Input: part model. Units: mm. Frame: model coordinates. Face numbers are marked on the shaded views. A direction names the side the tool comes from. Give positions to 0.01 mm unless a question says otherwise; leave off trailing zeros. Loops run counter-clockwise (first coordinate to the right, second up) from the corner with the lowest first, then second, coordinate; pieces in that order, holes last. Notation, with made-up numbers: M -19.75,20 L 32.25,20 A27 ccw 32.25,43 Z; hole C 64.5,75.25 d4. An arc over 180 degrees is marked long. Return JSON: item names as keys, results as strings. Group by question number.
```python
from build123d import *
from build123d import SkipClean  # not in build123d's __all__

# Parameters (mm, degrees)
F4_DEPTH = 10


with BuildPart() as f1:
    # F0 (on Front) → F1 (revolve)
    with BuildSketch(Plane.XZ):
        with BuildLine():
            Line((0, 5), (0, 0))
            Line((0, 0), (17.5, 0))
            Line((17.5, 0), (48.9644660941, 31.4644660941))
            ThreePointArc((48.9644660941, 31.4644660941), (46.4644660941, 32.5), (45.4289321881, 35))
            Line((45.4289321881, 35), (15.4289321881, 5))
            Line((15.4289321881, 5), (0, 5))
        make_face()
        with BuildLine():
            Line((45.4289321881, 35), (52.5, 35))
            ThreePointArc((52.5, 35), (48.9644660941, 38.5355339059), (45.4289321881, 35))
        make_face()
        with BuildLine():
            ThreePointArc((45.4289321881, 35), (46.4644660941, 32.5), (48.9644660941, 31.4644660941))
            Line((48.9644660941, 31.4644660941), (52.5, 35))
            Line((52.5, 35), (45.4289321881, 35))
        make_face()
    revolve(axis=Axis((0, 0, 17.5), (0, 0, 1)))

    # F2 (on face) → F3 (join, up to the next surface of F1)
    with BuildSketch(Plane(origin=(0, 0, 0), x_dir=(1, 0, 0), z_dir=(0, 0, -1))):
        with BuildLine():
            ThreePointArc((17.2839285714, -2.7414983381), (19.3665882743, -2.0194920684), (20.25, 0))
            ThreePointArc((20.25, 0), (19.3665882743, 2.0194920684), (17.2839285714, 2.7414983381))
            ThreePointArc((17.2839285714, 2.7414983381), (17.4458985151, 1.375), (17.5, 0))
            ThreePointArc((17.5, 0), (17.4458985151, -1.375), (17.2839285714, -2.7414983381))
        make_face()
        with BuildLine():
            ThreePointArc((-2.7414983381, 17.2839285714), (0, 17.5), (2.7414983381, 17.2839285714))
            ThreePointArc((2.7414983381, 17.2839285714), (2.7478737625, 17.3918806903), (2.75, 17.5))
            ThreePointArc((2.75, 17.5), (-0.1081193097, 20.2478737625), (-2.7414983381, 17.2839285714))
        make_face()
        with BuildLine():
            ThreePointArc((-2.7414983381, 17.2839285714), (0, 14.75), (2.7414983381, 17.2839285714))
            ThreePointArc((2.7414983381, 17.2839285714), (0, 17.5), (-2.7414983381, 17.2839285714))
        make_face()
        with BuildLine():
            ThreePointArc((2.75, -17.5), (2.7478737625, -17.3918806903), (2.7414983381, -17.2839285714))
            ThreePointArc((2.7414983381, -17.2839285714), (0, -17.5), (-2.7414983381, -17.2839285714))
            ThreePointArc((-2.7414983381, -17.2839285714), (-0.1081193097, -20.2478737625), (2.75, -17.5))
        make_face()
        with BuildLine():
            ThreePointArc((-17.2839285714, -2.7414983381), (-17.5, 0), (-17.2839285714, 2.7414983381))
            ThreePointArc((-17.2839285714, 2.7414983381), (-20.25, 0), (-17.2839285714, -2.7414983381))
        make_face()
    extrude(until=Until.NEXT, dir=(0, 0, 1))

    # F2 (on face) → F4 (join)
    with BuildSketch(Plane(origin=(0, 0, 0), x_dir=(1, 0, 0), z_dir=(0, 0, -1))):
        with BuildLine():
            ThreePointArc((17.2839285714, -2.7414983381), (19.3665882743, -2.0194920684), (20.25, 0))
            ThreePointArc((20.25, 0), (19.3665882743, 2.0194920684), (17.2839285714, 2.7414983381))
            ThreePointArc((17.2839285714, 2.7414983381), (17.4458985151, 1.375), (17.5, 0))
            ThreePointArc((17.5, 0), (17.4458985151, -1.375), (17.2839285714, -2.7414983381))
        make_face()
        with BuildLine():
            ThreePointArc((-2.7414983381, 17.2839285714), (0, 14.75), (2.7414983381, 17.2839285714))
            ThreePointArc((2.7414983381, 17.2839285714), (0, 17.5), (-2.7414983381, 17.2839285714))
        make_face()
        with BuildLine():
            ThreePointArc((-17.2839285714, -2.7414983381), (-17.5, 0), (-17.2839285714, 2.7414983381))
            ThreePointArc((-17.2839285714, 2.7414983381), (-20.25, 0), (-17.2839285714, -2.7414983381))
        make_face()
        with BuildLine():
            ThreePointArc((2.75, -17.5), (2.7478737625, -17.3918806903), (2.7414983381, -17.2839285714))
            ThreePointArc((2.7414983381, -17.2839285714), (0, -17.5), (-2.7414983381, -17.2839285714))
            ThreePointArc((-2.7414983381, -17.2839285714), (-0.1081193097, -20.2478737625), (2.75, -17.5))
        make_face()
        with BuildLine():
            ThreePointArc((-14.75, 0), (-15.4805079316, 1.8665882743), (-17.2839285714, 2.7414983381))
            ThreePointArc((-17.2839285714, 2.7414983381), (-17.5, 0), (-17.2839285714, -2.7414983381))
            ThreePointArc((-17.2839285714, -2.7414983381), (-15.4805079316, -1.8665882743), (-14.75, 0))
        make_face()
        with BuildLine():
            ThreePointArc((-2.7414983381, -17.2839285714), (0, -17.5), (2.7414983381, -17.2839285714))
            ThreePointArc((2.7414983381, -17.2839285714), (0, -14.75), (-2.7414983381, -17.2839285714))
        make_face()
        with BuildLine():
            ThreePointArc((-2.7414983381, 17.2839285714), (0, 17.5), (2.7414983381, 17.2839285714))
            ThreePointArc((2.7414983381, 17.2839285714), (2.7478737625, 17.3918806903), (2.75, 17.5))
            ThreePointArc((2.75, 17.5), (-0.1081193097, 20.2478737625), (-2.7414983381, 17.2839285714))
        make_face()
        with BuildLine():
            ThreePointArc((17.5, 0), (17.4458985151, 1.375), (17.2839285714, 2.7414983381))
            ThreePointArc((17.2839285714, 2.7414983381), (14.75, 0), (17.2839285714, -2.7414983381))
            ThreePointArc((17.2839285714, -2.7414983381), (17.4458985151, -1.375), (17.5, 0))
        make_face()
    with SkipClean():  # cleaning this boolean's faces spoils the solid; the shape is the same uncleaned
        extrude(amount=F4_DEPTH)


solid = f1.part
```
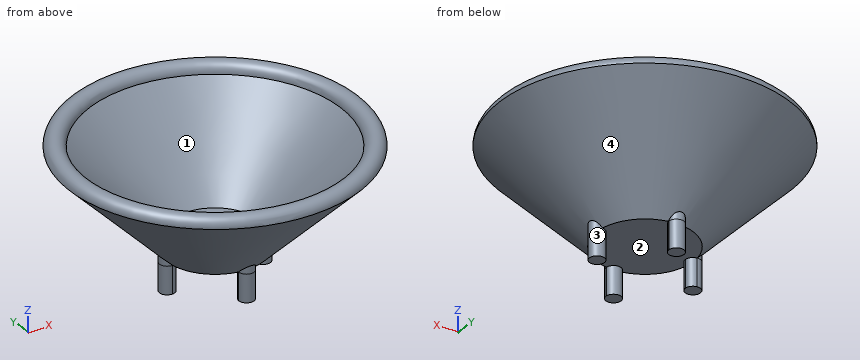
Item 1: First-contact query: pin 1 Ø6 at (x, y) = (-27, 31) entering from +Z; pin 2 Ø10.5 at (x, y) = (-4.5, 0.5) entering from -Z; pin 3 Ø5 at (y, z) = (-7.5, 30) entering from +X; pin 4 Ø4 at (y, z) = (-5, -3) entering from +X. Flat tips, straight axial feed; report the tip coordinate or a pass-through.
Item 2: Reachability of the marked faces 1 and 2 from +Z, -Z, +X, -X, +Y, -Y: full face, straight path, thin tool, end or side. Return the list, or none.
Item 3: Pull-direction query (X, two-part tool) for the marked faces 3 and 4; classes: pulls with the +X half, pulls with the -X half, needs draft (parallel to the pull), parting line crosses it, or undercut.
Item 4: Section B-B, the plane z = 27. Return loops of the section in (x, y), then the cut area to 3 significant figures.
Item 5: Section A-A, the plane x = 0. Return loops of the section in (y, z).
Item 6: Section C-C, the plane z = 19.5. Return loops of the section in (x, y), then the cut area to 3 significant figures.
Item 7: Material intervals for line 1 (X direction, y = -1.5, z = 35); line 2 (X direction, y = 19.5, z = 31); line 3 (Y direction, x = 31.5, z = 34.5), sorted ascending. Write a range as from..to.
Answer below:
{
 "1": {"pin 1": "z = 33.68", "pin 2": "z = 0", "pin 3": "x = 49.46", "pin 4": "through"},
 "2": {"face 1": "+Z", "face 2": "-Z"},
 "3": {"face 3": "undercut", "face 4": "parting line crosses it"},
 "4": {"outline": "C 0,0 d89; hole C 0,0 d74.86", "area": "1,820 mm^2"},
 "5": {"outline": "M -52.5,35 L -20.25,2.75 L -20.25,-10 L -14.75,-10 L -14.75,0 L 14.75,0 L 14.75,-10 L 20.25,-10 L 20.25,2.75 L 52.5,35 A3.54 ccw 45.43,35 L 15.43,5 L -15.43,5 L -45.43,35 A3.54 ccw Z"},
 "6": {"outline": "C 0,0 d74; hole C 0,0 d59.86", "area": "1,490 mm^2"},
 "7": {"line 1": "-52.48..-45.4, 45.4..52.48", "line 2": "-44.41..-36.55, 36.55..44.41", "line 3": "-41.37..-32.04, 32.04..41.37"}
}
